Part model, mm, in its own coordinate system. Face numbers are marked on the shaded views. A direction names the side the tool comes from. Round coordinates to 2 decimals unless told otherwise and drop trailing zeros. Write each loop counter-clockwise with the first axis right and the second up, starting at its lowest first coordinate (ties: lowest second). Pieces come first, ordered by that corner, then holes.
1) Saw through at A-A on y = 3.35. Write the cut outline in (x, z).
2) Flat gauge pins, fed straight in: pin 1 (1.5 mm diameter, centred on y = 2.5, z = -19.5, fed in from -X); pin 2 (4 mm diameter, centred on x = 13.5, z = -16, fed in from +Y); pin 3 (1.5 mm diameter, centred on y = 3.5, z = -3, fed in from +X). Where does each tip first touch, or does it go through?
3) Saw through at C-C on x = 11.75. Write the cut outline in (y, z), and give its area (3 significant figures).
4) Drill centre lines: L1, parallel to Z at x = 1.5, y = 0.6; L2, parallel to Z at x = 6.25, y = 2.6; L3, parallel to Y at x = 1.75, z = -20. Where is each one in solid material? Low to high.
5) Saw through at B-B on z = -15. Write the cut outline in (x, y), and give its area (3 significant figures).
6) Saw through at D-D on x = 6.75. Write the cut outline in (y, z).
7) Which spindle directions (+Z, -Z, +X, -X, +Y, -Y) get a long thin tool onto all of the face, cutting with end or side? Do the marked faces 1, 2, 3 and 4. Say none if no direction does.
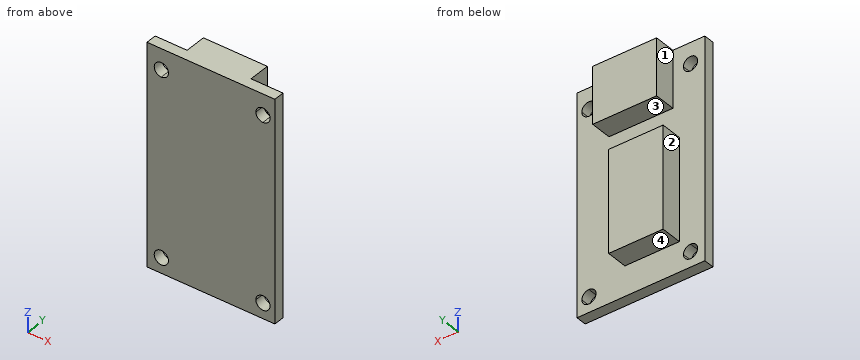
```python
from build123d import *

# Parameters (mm, degrees)
SKETCH1_W           = 9
SKETCH1_H           = 8
BOSS_EXTRUDE1_DEPTH = 1.5
SKETCH1_3_W         = 9
SKETCH1_3_H         = 8
BOSS_EXTRUDE2_DEPTH = 4.5
SKETCH2_W           = 7.673510846
SKETCH2_H           = 14.355500628
BOSS_EXTRUDE3_DEPTH = 3
CUT_EXTRUDE1_DEPTH  = 10


with BuildPart() as part:
    # Sketch1 → Boss-Extrude1 (new body)
    with BuildSketch(Plane(origin=(0, 0, 0), x_dir=(1, 0, 0), z_dir=(0, 1, 0))):
        Polygon((0, 31), (0, 0), (4.5, 0), (4.5, 8), (13.5, 8), (13.5, 0), (18, 0), (18, 31), align=None)
        with Locations((9, 4)):
            Rectangle(SKETCH1_W, SKETCH1_H)
    extrude(amount=BOSS_EXTRUDE1_DEPTH)

    # Sketch1<3> → Boss-Extrude2 (add)
    with BuildSketch(Plane(origin=(0, 0, 0), x_dir=(1, 0, 0), z_dir=(0, 1, 0))):
        with Locations((9, 4)):
            Rectangle(SKETCH1_3_W, SKETCH1_3_H)
    extrude(amount=BOSS_EXTRUDE2_DEPTH)

    # Sketch2 → Boss-Extrude3 (add)
    with BuildSketch(Plane(origin=(0, 1.5, 0), x_dir=(1, 0, 0), z_dir=(0, 1, 0))):
        with Locations((7.420466752, 19.616967898)):
            Rectangle(SKETCH2_W, SKETCH2_H)
    extrude(amount=BOSS_EXTRUDE3_DEPTH)

    # Sketch3 → Cut-Extrude1 (cut)
    with BuildSketch(Plane(origin=(0, 1.5, 0), x_dir=(1, 0, 0), z_dir=(0, 1, 0))):
        with BuildLine():
            ThreePointArc((3.017303644, 2.926927408), (2.724410426, 3.634034189), (2.017303644, 3.926927408))
            Line((2.017303644, 3.926927408), (2.017303644, 2.926927408))
            Line((2.017303644, 2.926927408), (3.017303644, 2.926927408))
        make_face()
        with BuildLine():
            Line((2.017303644, 2.926927408), (2.017303644, 3.926927408))
            ThreePointArc((2.017303644, 3.926927408), (1.310196863, 2.219820627), (3.017303644, 2.926927408))
            Line((3.017303644, 2.926927408), (2.017303644, 2.926927408))
        make_face()
        with BuildLine():
            ThreePointArc((17.320228506, 2.926927408), (17.027335287, 3.634034189), (16.320228506, 3.926927408))
            Line((16.320228506, 3.926927408), (16.320228506, 2.926927408))
            Line((16.320228506, 2.926927408), (15.320228506, 2.926927408))
            ThreePointArc((15.320228506, 2.926927408), (16.320228506, 1.926927408), (17.320228506, 2.926927408))
        make_face()
        with BuildLine():
            Line((16.320228506, 2.926927408), (16.320228506, 3.926927408))
            ThreePointArc((16.320228506, 3.926927408), (15.613121724, 3.634034189), (15.320228506, 2.926927408))
            Line((15.320228506, 2.926927408), (16.320228506, 2.926927408))
        make_face()
        with BuildLine():
            Line((2.017303644, 27.83251993), (2.017303644, 28.83251993))
            Line((2.017303644, 28.83251993), (3.017303644, 28.83251993))
            ThreePointArc((3.017303644, 28.83251993), (1.310196863, 29.539626711), (2.017303644, 27.83251993))
        make_face()
        with BuildLine():
            Line((3.017303644, 28.83251993), (2.017303644, 28.83251993))
            Line((2.017303644, 28.83251993), (2.017303644, 27.83251993))
            ThreePointArc((2.017303644, 27.83251993), (2.724410426, 28.125413148), (3.017303644, 28.83251993))
        make_face()
        with BuildLine():
            ThreePointArc((17.320228506, 28.83251993), (16.320228506, 29.83251993), (15.320228506, 28.83251993))
            Line((15.320228506, 28.83251993), (16.320228506, 28.83251993))
            Line((16.320228506, 28.83251993), (16.320228506, 27.83251993))
            ThreePointArc((16.320228506, 27.83251993), (17.027335287, 28.125413148), (17.320228506, 28.83251993))
        make_face()
        with BuildLine():
            Line((16.320228506, 28.83251993), (15.320228506, 28.83251993))
            ThreePointArc((15.320228506, 28.83251993), (15.613121724, 28.125413148), (16.320228506, 27.83251993))
            Line((16.320228506, 27.83251993), (16.320228506, 28.83251993))
        make_face()
    extrude(amount=-CUT_EXTRUDE1_DEPTH, mode=Mode.SUBTRACT)


solid = part.part
```
Completed:
1. outline: (3.58, -26.79) - (11.26, -26.79) - (11.26, -12.44) - (3.58, -12.44) - close; (4.5, -8) - (13.5, -8) - (13.5, 0) - (4.5, 0) - close
2. pin 1: stops at x = 3.58
2. pin 2: stops at y = 1.5
2. pin 3: stops at x = 13.5
3. outline: (0, -31) - (1.5, -31) - (1.5, -8) - (4.5, -8) - (4.5, 0) - (0, 0) - close
3. area: 70.5 mm2
4. L1: z = -31 to -29.69, -27.98 to -3.78, -2.07 to 0
4. L2: z = -26.79 to -12.44, -8 to 0
4. L3: y = 0 to 1.5
5. outline: (0, 0) - (18, 0) - (18, 1.5) - (11.26, 1.5) - (11.26, 4.5) - (3.58, 4.5) - (3.58, 1.5) - (0, 1.5) - close
5. area: 50.0 mm2
6. outline: (0, -31) - (1.5, -31) - (1.5, -26.79) - (4.5, -26.79) - (4.5, -12.44) - (1.5, -12.44) - (1.5, -8) - (4.5, -8) - (4.5, 0) - (0, 0) - close
7. face 1: +Z, -X, +Y
7. face 2: +Z, -Z, -X, +Y
7. face 3: +X, -X, +Y
7. face 4: -Z, +X, -X, +Y
